For this review, take the finished solid that the model builds, in its own axes (mm). Give positions to 0.01 mm unless a question says otherwise; leave off trailing zeros. Loops run counter-clockwise (first coordinate to the right, second up) from the corner with the lowest first, then second, coordinate; pieces in that order, holes last. Notation, with made-up numbers: (75, 33) -> (113, 33) arc R6 ccw to (113, 38) -> close; hole circle Ø8 at (10.25, 22.25). An arc over 180 degrees is marked (long way). One line per question, with ' | ' between items. Start each with the question number.
(1) Insertion check: P1, Ø1, axis at x = 2.5, z = -4.5, coming from the -Y side. The pin has a flat end and moves straight along its axis. Give the tip position at first contact, or say it passes through.
(2) Draft analysis for pull direction Z (two halves, no side actions). For faces 1 (the flat face through (2, 28.575, 1)), 2 (the cylindrical face through (1.57, -38.09, -0.84)), 3 (the flat face through (2, 14, 38.1)), 4 (the cylindrical face through (1.61, -31.6, 1.38)), state which applies: +Z half, -Z half, draft (parallel to the pull), parting line (faces both ways), or undercut.
(3) Consider section B-B (x = 1.45). Write out the cut boundary in (y, z) (3 decimals).
(4) Wall thickness on probe 1 along Y at (x, z) = (1.85, 0) (3 decimals); probe 2 along Z at (x, y) = (1.8, -22.5); probe 3 along Z at (x, y) = (2.65, -1): over which ranges is each line inside the solid? List them lowest first.
(5) Consider section D-D (z = 32). Write out the cut boundary in (x, y) (3 decimals), and give its area (3 significant figures).
(6) Consider section A-A (z = 0). Write out the cut boundary in (x, y) (3 decimals), and give its area (3 significant figures).
(7) Consider section C-C (y = -25.4). Write out the cut boundary in (x, z) (3 decimals).
from build123d import *

# Parameters (mm, degrees)
BOSS_EXTRUDE1_DEPTH = 3.175
SKETCH2_R           = 6.35
CUT_EXTRUDE1_DEPTH  = 54.975


with BuildPart() as part:
    # Sketch1 → Boss-Extrude1 (new body)
    with BuildSketch(Plane(origin=(0, 0, 0), x_dir=(0, 0, -1), z_dir=(1, 0, 0))):
        with BuildLine():
            Line((-38.1, 0), (-38.1, 28.575))
            Line((-38.1, 28.575), (38.1, 28.575))
            Line((38.1, 28.575), (38.1, 0))
            ThreePointArc((38.1, 0), (0, -38.1), (-38.1, 0))
        make_face()
    extrude(amount=BOSS_EXTRUDE1_DEPTH)

    # Sketch2 → Cut-Extrude1 (cut, through all)
    with BuildSketch(Plane(origin=(3.175, 0, 0), x_dir=(0, 0, -1), z_dir=(1, 0, 0))):
        with Locations((0, -25.4)):
            Circle(SKETCH2_R)
    extrude(amount=-CUT_EXTRUDE1_DEPTH, mode=Mode.SUBTRACT)


solid = part.part
A:
1) P1: stops at y = -37.89
2) face 1: draft | face 2: parting line | face 3: +Z half | face 4: undercut
3) outline: (0, -38.1) -> (28.575, -38.1) -> (28.575, 38.1) -> (0, 38.1) arc R38.1 ccw to start; hole circle Ø12.7 at (-25.4, 0)
4) probe 1: y = -38.1 to -31.75, -19.05 to 28.575 | probe 2: z = -30.75 to -5.65, 5.65 to 30.75 | probe 3: z = -38.09 to 38.09
5) outline: (0, -20.679) -> (3.175, -20.679) -> (3.175, 28.575) -> (0, 28.575) -> close | area: 156 mm^2
6) outline: (0, -38.1) -> (3.175, -38.1) -> (3.175, -31.75) -> (0, -31.75) -> close; (0, -19.05) -> (3.175, -19.05) -> (3.175, 28.575) -> (0, 28.575) -> close | area: 171 mm^2
7) outline: (0, -28.398) -> (3.175, -28.398) -> (3.175, -6.35) -> (0, -6.35) -> close; (0, 6.35) -> (3.175, 6.35) -> (3.175, 28.398) -> (0, 28.398) -> close
